Read the model definition and answer for the solid it produces. Units are mm, in the model's axes. Give positions to 0.01 mm unless a question says otherwise; leave off trailing zeros. Order: outer loops, then holes, each group sorted by start corner. A loop starts at its lowest first (then second) coordinate and runs counter-clockwise, first axis right, second up. Notation, with made-up numbers: M 82,21 L 122,21 A12 ccw 122,25 Z; hole C 51.5,-26 d11. An arc over 180 degrees is marked long. One line per item, written item: value. Start each with the question number.
from build123d import *

# Parameters (mm, degrees)
SKETCH1_W               = 96
SKETCH1_H               = 5
SKETCH2_R               = 1.25
CUT_EXTRUDE1_DEPTH      = 56
CUT_EXTRUDE1_DEPTH_BACK = 56
SKETCH4_R               = 1.25
CUT_EXTRUDE2_DEPTH      = 56.0000001
CUT_EXTRUDE2_DEPTH_BACK = 56.0000001
SKETCH5_R               = 1.25
CUT_EXTRUDE3_DEPTH      = 5
CIRPATTERN1_COUNT       = 4


with BuildPart() as part:
    # Sketch1 → Revolve1 (revolve)
    with BuildSketch(Plane.XY):
        with Locations((48, 52.5)):
            Rectangle(SKETCH1_W, SKETCH1_H)
    revolve(axis=Axis((0, 0, 0), (1, 0, 0)))

    # Sketch2 → Cut-Extrude1 (cut, two sides)
    with BuildSketch(Plane(origin=(0, 0, 0), x_dir=(1, 0, 0), z_dir=(0, 1, 0))) as cut_extrude1_sk:
        with Locations((93.637235836, 0)):
            Circle(SKETCH2_R)
    extrude(amount=CUT_EXTRUDE1_DEPTH, mode=Mode.SUBTRACT)
    extrude(cut_extrude1_sk.sketch, amount=-CUT_EXTRUDE1_DEPTH_BACK, mode=Mode.SUBTRACT)

    # Sketch4 → Cut-Extrude2 (cut, two sides)
    with BuildSketch(Plane.XY) as cut_extrude2_sk:
        with Locations((93.481477352, 0)):
            Circle(SKETCH4_R)
    extrude(amount=CUT_EXTRUDE2_DEPTH, mode=Mode.SUBTRACT)
    extrude(cut_extrude2_sk.sketch, amount=-CUT_EXTRUDE2_DEPTH_BACK, mode=Mode.SUBTRACT)

    # Sketch5 → Cut-Extrude3 (cut)
    with BuildSketch(Plane(origin=(96, 0, 0), x_dir=(0, 0, -1), z_dir=(1, 0, 0))):
        with Locations((0, 52.5)):
            Circle(SKETCH5_R)
    cut_extrude3 = extrude(amount=-CUT_EXTRUDE3_DEPTH, mode=Mode.SUBTRACT)

    # CirPattern1: Cut-Extrude3 ×4 about axis
    cirpattern1_axis = Axis((0, 0, 0), (1, 0, 0))
    for i in range(1, CIRPATTERN1_COUNT):
        add(cut_extrude3.rotate(cirpattern1_axis, i * 360 / CIRPATTERN1_COUNT), mode=Mode.SUBTRACT)


solid = part.part
Q1. Find section C-C, the plane x = 81.5. Give the vertices of the cut face in (y, z).
Q2. Each of these flat-tipped pins is pushed along its axis until it touches: pin 1 (3 mm diameter, centred on x = 47.5, y = 33, fed in from +Z); pin 2 (10 mm diameter, centred on x = 46, y = 31, fed in from +Z); pin 3 (6 mm diameter, centred on x = 13, y = 41, fed in from +Z). Where does it stop, or does it pass through?
Q3. Determine the mould class of faces 1 (the flat face through (0, -12, -49)), 2 (the cylindrical face through (48.672, -11.923, -53.692)), 3 (the cylindrical face through (48.67, 47.69, 15.02)) for opening direction Z: released by +Z, released by -Z, zero draft, split by the parting line, or undercut.
Q4. Consider probe 1 along Z at (x, y) = (92, 0); probe 2 along X at (y, z) = (0, 51). Determine where each line is inside the solid, lowest interval first.
Q5. Find section A-A, the plane y = 15.5. Give the vertices of the cut face in (x, z).
Q6. Find section B-B, the plane z = 44. Give the vertices of the cut face in (x, y).
Evaluation:
1. outline: C 0,0 d110; hole C 0,0 d100
2. pin 1: z = 45.09
2. pin 2: z = 48.47
2. pin 3: z = 39.76
3. face 1: zero draft
3. face 2: split by the parting line
3. face 3: undercut
4. probe 1: -55 to -53.75, -51.25 to -50, 50 to 51.25, 53.75 to 55
4. probe 2: 0 to 92.23, 94.73 to 96
5. outline: M 0,-52.77 L 96,-52.77 L 96,-47.54 L 0,-47.54 Z; M 0,47.54 L 96,47.54 L 96,52.77 L 0,52.77 Z
6. outline: M 0,-33 L 96,-33 L 96,-23.75 L 0,-23.75 Z; M 0,23.75 L 96,23.75 L 96,33 L 0,33 Z
